Autodesk Inventor part; units mm, degrees
ref_plane "YZ Plane" through (0, 0, 0) normal (1, 0, 0) x (0, 1, 0)
ref_plane "XZ Plane" through (0, 0, 0) normal (0, 1, 0) x (-1, 0, 0)
ref_plane "XY Plane" through (0, 0, 0) normal (0, 0, 1) x (1, 0, 0)
sketch "Sketch1" plane through (0, 0, 0) normal (1, 0, 0) x (0, 1, 0)
  line L0 (0, 45) -> (30, 45)
  line L1 (30, 45) -> (30, -45)
  line L2 (30, -45) -> (0, -45)
  line L3 (0, -45) -> (0, 45)
  line L4 (30, 42) -> (3, 42)
  line L5 (3, 42) -> (3, -42)
  line L6 (3, -42) -> (30, -42)
  line L7 (30, -42) -> (30, 42)
  point P0 (0, 0)
  point P1 (30, -42)
  dimension "d0" = 45
  dimension "d1" = 90
  dimension "d2" = 30
  dimension "d3" = 0
  dimension "d4" = 3
  dimension "d5" = 3
  dimension "d6" = 3
extrude "Extrusion1" add sketch "Sketch1" along normal blind 100 contours L0 L1 L4 L5 L6 L2 L3
sketch "Sketch2" plane through (100, 0, 0) normal (1, 0, 0) x (0, 0, -1)
  line L0 (-50, 0) -> (50, 0)
  line L1 (50, 0) -> (50, 100)
  line L2 (50, 100) -> (-50, 100)
  line L3 (-50, 100) -> (-50, 0)
  line L4 (-45, 0) -> (45, 0)
  point P0 (0, 0)
  point P1 (0, 0)
  dimension "d9" = 100
  dimension "d10" = 100
extrude "Extrusion2" add sketch "Sketch2" along normal blind 3
sketch "Sketch4" plane through (0, 0, 0) normal (0, 0, 1) x (1, 0, 0)
  line L0 (103, 100) -> (103, 0)
  line L1 (103, 70) -> (133, 70)
  line L2 (133, 70) -> (133, 40)
  line L3 (133, 40) -> (128, 40)
  line L4 (128, 40) -> (128, 65)
  line L5 (128, 65) -> (103, 65)
  line L6 (100, 100) -> (103, 100)
  point P0 (0, 0)
  point P1 (115.5, 65)
  point P2 (118, 70)
  point P3 (128, 52.5)
  point P4 (101.5, 100)
  dimension "d13" = 5
  dimension "d14" = 5
  dimension "d15" = 30
  dimension "d16" = 30
  dimension "d17" = 30
extrude "Extrusion3" add sketch "Sketch4" along normal mid plane 5
fillet "Fillet1" radius 2.5 8 edges at (118, 70, 2.5) (115.5, 65, 2.5) (133, 55, 2.5) (128, 52.5, 2.5) (133, 55, -2.5) (133, 70, 0) (118, 70, -2.5) (115.5, 65, -2.5)
equation "\"d5\" = d4"
equation "\"d6\" = d4"
equation "\"d10\" = d9"
equation "\"d16\" = d15"
properties part number "RS2_AshBucket"
Can you work these out from the model? Positions are in its coordinate system, mm. A direction names the side the tool comes from. Give positions to 0.01 mm unless a question says otherwise; leave off trailing zeros. Order: outer loops, then holes, each group sorted by start corner. A loop starts at its lowest first (then second) coordinate and runs counter-clockwise, first axis right, second up. Notation, with made-up numbers: M 13,65.5 L 34,65.5 A27 ccw 34,93.5 Z; hole C -14,-19.5 d1. An arc over 180 degrees is marked long. Write item = value, one per line. Start each with the question number.
Q1. Suppose I cut it at C-C (y = 12). Write out the boundary of the cut face in (x, z), plus the area to 3 significant figures.
Q2. Will these pins go through, and if not, where does the flat tip stop? pin 1 Ø1 at (y, z) = (31.5, 22) entering from +X; pin 2 Ø14 at (x, y) = (118.5, 53.5) entering from +Z; pin 3 Ø24 at (x, y) = (49, 10) entering from -Z; pin 4 Ø8 at (x, y) = (25.5, 19) entering from +Z.
Q3. For faces 1 (the flat face through (49, 16, -42)), 2 (the flat face through (131, 40, 0)), 3 (the flat face through (49, 15, 45)), which set-ups out of +Z, -Z, +X, -X, +Y, -Y let a thin tool reach every point of the face, with its end or its side?
Q4. Suppose I cut it at B-B (x = 57). Write out the boundary of the cut face in (y, z), plus the area to 3 significant figures.
Q5. I need wall thicknesses on probe 1 along Z at (x, y) = (86, 24.5); probe 2 along X at (y, z) = (44, 20.5); probe 3 along Y at (x, z) = (48, -30.5). Which ranges of each line are inside material? Lowest first, please. Write a range as [from, to].
Q6. Suppose I cut it at D-D (z = 5). Write out the boundary of the cut face in (x, y).
Q7. We'd pull the mould along Z, two halves only. Please class faces 4 (the flat face through (100, 51, 1)), 5 (the flat face through (129, 54, -2.5)), 6 (the flat face through (49, 3, 1)), 7 (the flat face through (49, 30, 44)): pulls with the +Z half, pulls with the -Z half, needs draft (parallel to the pull), parting line crosses it, or undercut.
Check result:
q1.outline = M 0,-45 L 100,-45 L 100,-50 L 103,-50 L 103,50 L 100,50 L 100,45 L 0,45 L 0,42 L 100,42 L 100,-42 L 0,-42 Z
q1.area = 900 mm2
q2.pin_1 = 103
q2.pin_2 = through
q2.pin_3 = -45
q2.pin_4 = 45
q3.face_1 = -X, +Y
q3.face_2 = +Z, -Z, +X, -Y
q3.face_3 = +Z, -X, +Y, -Y
q4.outline = M 0,-45 L 30,-45 L 30,-42 L 3,-42 L 3,42 L 30,42 L 30,45 L 0,45 Z
q4.area = 432 mm2
q5.probe_1 = [-45, -42], [42, 45]
q5.probe_2 = [100, 103]
q5.probe_3 = [0, 3]
q6.outline = M 0,0 L 103,0 L 103,100 L 100,100 L 100,3 L 0,3 Z
q7.face_4 = undercut
q7.face_5 = pulls with the -Z half
q7.face_6 = undercut
q7.face_7 = needs draft
